from build123d import *

# Parameters (mm, degrees)
F1_DEPTH = 1
F2_DEPTH = 3
F3_DEPTH = 0.7


with BuildPart() as f1:
    # F0 (on Top) → F1 (new body)
    with BuildSketch(Plane.XY):
        with BuildLine():
            ThreePointArc((-69.95, 5), (-69.776457, 5.355066), (-69.389682, 5.436268))
            ThreePointArc((-69.389682, 5.436268), (-69.10934, 10.224685), (-68.657801, 15))
            Line((-68.657801, 15), (-71.5, 15))
            Line((-71.5, 15), (-71.5, 0))
            Line((-71.5, 0), (-69.95, 0))
            Line((-69.95, 0), (-69.95, 5))
        make_face()
        with BuildLine():
            ThreePointArc((-69.05, 5), (-69.144934, 5.276457), (-69.389682, 5.436268))
            ThreePointArc((-69.389682, 5.436268), (-69.776457, 5.355066), (-69.95, 5))
            Line((-69.95, 5), (-69.95, 0))
            Line((-69.95, 0), (-71.5, 0))
            ThreePointArc((-71.5, 0), (0, -71.5), (71.5, 0))
            Line((71.5, 0), (69.95, 0))
            Line((69.95, 0), (69.95, 5))
            ThreePointArc((69.95, 5), (69.776457, 5.355066), (69.389682, 5.436268))
            ThreePointArc((69.389682, 5.436268), (69.144934, 5.276457), (69.05, 5))
            Line((69.05, 5), (69.05, 0))
            Line((69.05, 0), (64.5, 0))
            Line((64.5, 0), (64.5, 15))
            Line((64.5, 15), (-64.5, 15))
            Line((-64.5, 15), (-64.5, 0))
            Line((-64.5, 0), (-69.05, 0))
            Line((-69.05, 0), (-69.05, 5))
        make_face()
        with BuildLine():
            Line((69.95, 0), (71.5, 0))
            Line((71.5, 0), (71.5, 15))
            Line((71.5, 15), (68.657801, 15))
            ThreePointArc((68.657801, 15), (69.10934, 10.224685), (69.389682, 5.436268))
            ThreePointArc((69.389682, 5.436268), (69.776457, 5.355066), (69.95, 5))
            Line((69.95, 5), (69.95, 0))
        make_face()
        with BuildLine():
            ThreePointArc((-68.657801, 15), (-69.10934, 10.224685), (-69.389682, 5.436268))
            ThreePointArc((-69.389682, 5.436268), (-69.144934, 5.276457), (-69.05, 5))
            Line((-69.05, 5), (-69.05, 0))
            Line((-69.05, 0), (-64.5, 0))
            Line((-64.5, 0), (-64.5, 15))
            Line((-64.5, 15), (-68.657801, 15))
        make_face()
        with BuildLine():
            Line((68.657801, 15), (64.5, 15))
            Line((64.5, 15), (64.5, 0))
            Line((64.5, 0), (69.05, 0))
            Line((69.05, 0), (69.05, 5))
            ThreePointArc((69.05, 5), (69.144934, 5.276457), (69.389682, 5.436268))
            ThreePointArc((69.389682, 5.436268), (69.10934, 10.224685), (68.657801, 15))
        make_face()
    extrude(amount=F1_DEPTH)

    # F0 (on Top) → F2 (join)
    with BuildSketch(Plane.XY):
        with BuildLine():
            Line((69.95, 0), (71.5, 0))
            Line((71.5, 0), (71.5, 15))
            Line((71.5, 15), (68.657801, 15))
            ThreePointArc((68.657801, 15), (69.10934, 10.224685), (69.389682, 5.436268))
            ThreePointArc((69.389682, 5.436268), (69.776457, 5.355066), (69.95, 5))
            Line((69.95, 5), (69.95, 0))
        make_face()
        with BuildLine():
            ThreePointArc((-69.95, 5), (-69.776457, 5.355066), (-69.389682, 5.436268))
            ThreePointArc((-69.389682, 5.436268), (-69.10934, 10.224685), (-68.657801, 15))
            Line((-68.657801, 15), (-71.5, 15))
            Line((-71.5, 15), (-71.5, 0))
            Line((-71.5, 0), (-69.95, 0))
            Line((-69.95, 0), (-69.95, 5))
        make_face()
        with BuildLine():
            ThreePointArc((-68.657801, 15), (-69.10934, 10.224685), (-69.389682, 5.436268))
            ThreePointArc((-69.389682, 5.436268), (-69.144934, 5.276457), (-69.05, 5))
            Line((-69.05, 5), (-69.05, 0))
            Line((-69.05, 0), (-64.5, 0))
            Line((-64.5, 0), (-64.5, 15))
            Line((-64.5, 15), (-68.657801, 15))
        make_face()
        with BuildLine():
            Line((68.657801, 15), (64.5, 15))
            Line((64.5, 15), (64.5, 0))
            Line((64.5, 0), (69.05, 0))
            Line((69.05, 0), (69.05, 5))
            ThreePointArc((69.05, 5), (69.144934, 5.276457), (69.389682, 5.436268))
            ThreePointArc((69.389682, 5.436268), (69.10934, 10.224685), (68.657801, 15))
        make_face()
    extrude(amount=-F2_DEPTH)

    # F0 (on Top) → F3 (cut)
    with BuildSketch(Plane.XY):
        with BuildLine():
            ThreePointArc((-68.657801, 15), (-69.10934, 10.224685), (-69.389682, 5.436268))
            ThreePointArc((-69.389682, 5.436268), (-69.144934, 5.276457), (-69.05, 5))
            Line((-69.05, 5), (-69.05, 0))
            Line((-69.05, 0), (-64.5, 0))
            Line((-64.5, 0), (-64.5, 15))
            Line((-64.5, 15), (-68.657801, 15))
        make_face()
        with BuildLine():
            Line((68.657801, 15), (64.5, 15))
            Line((64.5, 15), (64.5, 0))
            Line((64.5, 0), (69.05, 0))
            Line((69.05, 0), (69.05, 5))
            ThreePointArc((69.05, 5), (69.144934, 5.276457), (69.389682, 5.436268))
            ThreePointArc((69.389682, 5.436268), (69.10934, 10.224685), (68.657801, 15))
        make_face()
    extrude(amount=-F3_DEPTH, mode=Mode.SUBTRACT)


solid = f1.part
Design review of the part built by this model. Coordinates are the model's own, in mm. A direction names the side the tool comes from. Coordinates: 2 decimals unless noted, no trailing zeros. Loops run counter-clockwise (first coordinate to the right, second up) from the corner with the lowest first, then second, coordinate; pieces in that order, holes last. Notation, with made-up numbers: (54, 42) -> (99, 42) arc R4 cw to (99, 49) -> close; hole circle Ø8 at (10.25, 85). An arc over 180 degrees is marked (long way). Use a Markdown table: item, result. Add a question column.
Item 1: We need section A-A, the plane x = 0. Write out the cut boundary in (y, z).
Item 2: Wall thickness on L1, parallel to X at y = 4.5, z = -2.55; L2, parallel to X at y = 9, z = -1.15; L3, parallel to Z at x = 54, y = 3.5: over which ranges is each line inside the solid? List them lowest first. Write a range as from..to.
Item 3: The part is to be moulded in two halves that separate along X. For faces 1 (the flat face through (-71.5, 8, -1)), 2 (the flat face through (-69.95, 2, -1)), 3 (the flat face through (-68, 8, -3)), say which applies: +X half, -X half, draft (parallel to the pull), parting line (faces both ways), or undercut.
Item 4: Clearance check with flat-ended pins moving along their axes: P1, Ø1.2, axis at x = -70.5, z = -1, coming from the -Y side; P2, Ø2, axis at y = -51.5, z = -1.5, coming from the -X side; P3, Ø2, axis at y = -19, z = -0.5, coming from the -X side; P4, Ø10, axis at x = -54, y = -17, coming from the -Z side. State where each tip first meets the part, or that it passes through.
Item 5: Machinability: for faces 4 (the flat face through (69.95, 3, -1)), 5 (the flat face through (-1, -18, 1)), which of the approach directions +Z, -Z, +X, -X, +Y, -Y give a long, thin tool a straight path to every point of the face, cutting with its end or side? Answer none if there is none.
Item 6: We need section B-B, the plane y = -39. Write out the cut boundary in (x, z), and give its area (3 significant figures).
Numbers:
| question | item | result |
|---|---|---|
| 1 | outline | (-71.5, 0) -> (15, 0) -> (15, 1) -> (-71.5, 1) -> close |
| 2 | L1 | x = -71.5..-69.95, -69.05..-64.5, 64.5..69.05, 69.95..71.5 |
| 2 | L2 | x = -71.5..-64.5, 64.5..71.5 |
| 2 | L3 | z = 0..1 |
| 3 | face 1 | -X half |
| 3 | face 2 | undercut |
| 3 | face 3 | draft |
| 4 | P1 | stops at y = 0 |
| 4 | P2 | passes through |
| 4 | P3 | stops at x = -69.16 |
| 4 | P4 | stops at z = 0 |
| 5 | face 4 | -Z, -Y |
| 5 | face 5 | +Z, +X, -X, +Y, -Y |
| 6 | outline | (-59.93, 0) -> (59.93, 0) -> (59.93, 1) -> (-59.93, 1) -> close |
| 6 | area | 120 mm^2 |
